```python
from build123d import *

# Parameters (mm, degrees)
SKETCH1_W           = 88
SKETCH1_H           = 68
BOSS_EXTRUDE1_DEPTH = 5.588
SKETCH2_R           = 1.8
CUT_EXTRUDE1_DEPTH  = 94.929750833


with BuildPart() as part:
    # Sketch1 → Boss-Extrude1 (new body)
    with BuildSketch(Plane(origin=(0, 0, 0), x_dir=(1, 0, 0), z_dir=(0, 1, 0))):
        with Locations((-43.165773612, -0.549967556)):
            Rectangle(SKETCH1_W, SKETCH1_H)
    extrude(amount=BOSS_EXTRUDE1_DEPTH)

    # Sketch2 → Cut-Extrude1 (cut, through all)
    with BuildSketch(Plane(origin=(0, 5.588, 0), x_dir=(1, 0, 0), z_dir=(0, 1, 0))):
        with Locations(Location((-68.165773612, 29.450032444, 0), (0, 0, 270))):
            Circle(SKETCH2_R)
        with Locations(Location((-43.165773612, 29.450032444, 0), (0, 0, 270))):
            Circle(SKETCH2_R)
        with Locations(Location((-18.165773612, 29.450032444, 0), (0, 0, 270))):
            Circle(SKETCH2_R)
        with Locations(Location((-43.165773612, -30.549967556, 0), (0, 0, 270))):
            Circle(SKETCH2_R)
        with Locations(Location((-68.165773612, -30.549967556, 0), (0, 0, 270))):
            Circle(SKETCH2_R)
        with Locations(Location((-18.165773612, -30.549967556, 0), (0, 0, 270))):
            Circle(SKETCH2_R)
        with Locations(Location((-62.965773612, -0.549967556, 0), (0, 0, 270))):
            Circle(SKETCH2_R)
        with Locations(Location((-23.365773612, -0.549967556, 0), (0, 0, 270))):
            Circle(SKETCH2_R)
        with Locations(Location((-23.365773612, -17.349967556, 0), (0, 0, 270))):
            Circle(SKETCH2_R)
        with Locations(Location((-23.365773612, 16.250032444, 0), (0, 0, 270))):
            Circle(SKETCH2_R)
        with Locations(Location((-62.965773612, -13.049967556, 0), (0, 0, 270))):
            Circle(SKETCH2_R)
        with Locations(Location((-62.965773612, 11.950032444, 0), (0, 0, 270))):
            Circle(SKETCH2_R)
        with Locations(Location((-82.645773612, 24.450032444, 0), (0, 0, 270))):
            Circle(SKETCH2_R)
        with Locations(Location((-3.685773612, 24.450032444, 0), (0, 0, 270))):
            Circle(SKETCH2_R)
        with Locations(Location((-82.645773612, 14.450032444, 0), (0, 0, 270))):
            Circle(SKETCH2_R)
        with Locations(Location((-3.685773612, 14.450032444, 0), (0, 0, 270))):
            Circle(SKETCH2_R)
        with Locations(Location((-82.645773612, 4.450032444, 0), (0, 0, 270))):
            Circle(SKETCH2_R)
        with Locations(Location((-3.685773612, 4.450032444, 0), (0, 0, 270))):
            Circle(SKETCH2_R)
        with Locations(Location((-82.645773612, -5.549967556, 0), (0, 0, 270))):
            Circle(SKETCH2_R)
        with Locations(Location((-3.685773612, -5.549967556, 0), (0, 0, 270))):
            Circle(SKETCH2_R)
        with Locations(Location((-82.645773612, -15.549967556, 0), (0, 0, 270))):
            Circle(SKETCH2_R)
        with Locations(Location((-3.685773612, -15.549967556, 0), (0, 0, 270))):
            Circle(SKETCH2_R)
        with Locations(Location((-82.645773612, -25.549967556, 0), (0, 0, 270))):
            Circle(SKETCH2_R)
        with Locations(Location((-3.685773612, -25.549967556, 0), (0, 0, 270))):
            Circle(SKETCH2_R)
    extrude(amount=-CUT_EXTRUDE1_DEPTH, mode=Mode.SUBTRACT)


solid = part.part
```
Geometry check sheet. Reference: the model listing, model coordinates, mm. Coordinates: 2 decimals unless noted, no trailing zeros. Loops run counter-clockwise (first coordinate to the right, second up) from the corner with the lowest first, then second, coordinate; pieces in that order, holes last.
Item 1: Release check for a two-part mould opening along Z. For faces 1 (the face through (-44, 5.588, 0)), 2 (the face through (-44.923, 2.833, -29.84)), 3 (the face through (-44, 3, -33.45)) record: released by +Z, released by -Z, zero draft, split by the parting line, or undercut.
Item 2: Thickness scan on line 1 (Z direction, x = -23.5, y = 0.3); line 2 (X direction, y = 0.9, z = -4.5); line 3 (X direction, y = 2.35, z = 6.5). Record the ranges inside material, lowest first.
Item 3: Sectioned sample at A-A, the plane y = 3. Count the separate pieces of the cut face and the enclosed holes in it, then the cut area to 3 significant figures.
Item 4: Sectioned sample at B-B, the plane z = 12.5. Record the boundary of the cut face in (x, y).
Check result:
1. face 1: zero draft
1. face 2: undercut
1. face 3: released by -Z
2. line 1: z = -33.45 to -18.05, -14.46 to -1.25, 2.34 to 15.55, 19.14 to 34.55
2. line 2: x = -87.17 to -84.45, -80.85 to -5.49, -1.89 to 0.83
2. line 3: x = -87.17 to -84.17, -81.12 to -5.21, -2.16 to 0.83
3. separate pieces: 1
3. enclosed holes: 24
3. area: 5,740 mm2
4. outline: (-87.17, 0) - (-64.68, 0) - (-64.68, 5.59) - (-87.17, 5.59) - close; (-61.25, 0) - (0.83, 0) - (0.83, 5.59) - (-61.25, 5.59) - close
